```python
from build123d import *

# Parameters (mm, degrees)
SKETCH1_W           = 200
SKETCH1_H           = 200
BOSS_EXTRUDE1_DEPTH = 5
SKETCH2_W           = 100
SKETCH2_H           = 100
CUT_EXTRUDE1_DEPTH  = 10
FILLET1_R           = 10
FILLET2_R           = 10
SKETCH3_R           = 3
CUT_EXTRUDE2_DEPTH  = 10
SKETCH4_R           = 1.5
CUT_EXTRUDE3_DEPTH  = 10
SKETCH5_W           = 210
SKETCH5_H           = 210
BOSS_EXTRUDE2_DEPTH = 5
FILLET3_R           = 10
CIRPATTERN1_COUNT   = 4
SKETCH6_OUTSIDE_W   = 271.406
SKETCH6_OUTSIDE_H   = 271.406
SKETCH6_OUTSIDE_W_2 = 55
SKETCH6_OUTSIDE_H_2 = 132
CUT_EXTRUDE4_DEPTH  = 10
SKETCH8_W           = 55
SKETCH8_H           = 30
BOSS_EXTRUDE3_DEPTH = 5
SKETCH9_R           = 3
CUT_EXTRUDE6_DEPTH  = 5
SKETCH11_W          = 55
SKETCH11_H          = 19
CUT_EXTRUDE7_DEPTH  = 39
FILLET6_R           = 5
SKETCH12_W          = 15
SKETCH12_H          = 75
CUT_EXTRUDE8_DEPTH  = 10
FILLET7_R           = 5


with BuildPart() as part:
    # Sketch1 → Boss-Extrude1 (new body)
    with BuildSketch(Plane(origin=(0, 0, 0), x_dir=(1, 0, 0), z_dir=(0, 1, 0))):
        with Locations((100, 100)):
            Rectangle(SKETCH1_W, SKETCH1_H)
    extrude(amount=BOSS_EXTRUDE1_DEPTH)

    # Sketch2 → Cut-Extrude1 (cut)
    with BuildSketch(Plane(origin=(0, 5, 0), x_dir=(1, 0, 0), z_dir=(0, 1, 0))):
        with Locations((100, 100)):
            Rectangle(SKETCH2_W, SKETCH2_H)
    extrude(amount=-CUT_EXTRUDE1_DEPTH, mode=Mode.SUBTRACT)

    # Fillet1
    fillet1_edges = [part.edges().sort_by_distance(p)[0] for p in [
        (150, 2.5, -150),
        (150, 2.5, -50),
        (50, 2.5, -50),
        (50, 2.5, -150),
    ]]
    fillet(fillet1_edges, radius=FILLET1_R)

    # Fillet2
    fillet2_edges = [part.edges().sort_by_distance(p)[0] for p in [
        (0, 2.5, -200),
        (200, 2.5, -200),
        (200, 2.5, 0),
        (0, 2.5, 0),
    ]]
    fillet(fillet2_edges, radius=FILLET2_R)

    # Sketch3 → Cut-Extrude2 (cut)
    with BuildSketch(Plane(origin=(0, 5, 0), x_dir=(1, 0, 0), z_dir=(0, 1, 0))):
        with Locations((10, 190)):
            Circle(SKETCH3_R)
        with Locations((190, 190)):
            Circle(SKETCH3_R)
        with Locations((190, 10)):
            Circle(SKETCH3_R)
        with Locations((10, 10)):
            Circle(SKETCH3_R)
    extrude(amount=-CUT_EXTRUDE2_DEPTH, mode=Mode.SUBTRACT)

    # Sketch4 → Cut-Extrude3 (cut)
    with BuildSketch(Plane(origin=(0, 5, 0), x_dir=(1, 0, 0), z_dir=(0, 1, 0))):
        with Locations((198, 126)):
            Circle(SKETCH4_R)
        with Locations((191, 126)):
            Circle(SKETCH4_R)
        with Locations((196.89, 142)):
            Circle(SKETCH4_R)
        with Locations((154.75, 48)):
            Circle(SKETCH4_R)
        with Locations((196.75, 48)):
            Circle(SKETCH4_R)
        with Locations((196.75, 24)):
            Circle(SKETCH4_R)
        with Locations((154.75, 24)):
            Circle(SKETCH4_R)
        with Locations((242.150033952, -166.330778193)):
            Circle(SKETCH4_R)
        with Locations((285.400033952, -64.330778193)):
            Circle(SKETCH4_R)
        with Locations((242.150033952, -142.330778193)):
            Circle(SKETCH4_R)
        with Locations((284.290033952, -48.330778193)):
            Circle(SKETCH4_R)
        with Locations((284.150033952, -142.330778193)):
            Circle(SKETCH4_R)
        with Locations((284.150033952, -166.330778193)):
            Circle(SKETCH4_R)
        with Locations((278.400033952, -64.330778193)):
            Circle(SKETCH4_R)
    cut_extrude3 = extrude(amount=-CUT_EXTRUDE3_DEPTH, mode=Mode.SUBTRACT)

    # Sketch5 → Boss-Extrude2 (add)
    with BuildSketch(Plane(origin=(0, 5, 0), x_dir=(1, 0, 0), z_dir=(0, 1, 0))):
        with Locations((100, 100)):
            Rectangle(SKETCH5_W, SKETCH5_H)
        with BuildLine():
            Line((0, 190), (0, 10))
            ThreePointArc((0, 10), (2.928932188, 2.928932188), (10, 0))
            Line((10, 0), (190, 0))
            ThreePointArc((190, 0), (197.071067812, 2.928932188), (200, 10))
            Line((200, 10), (200, 190))
            ThreePointArc((200, 190), (197.071067812, 197.071067812), (190, 200))
            Line((190, 200), (10, 200))
            ThreePointArc((10, 200), (2.928932188, 197.071067812), (0, 190))
        make_face(mode=Mode.SUBTRACT)
    extrude(amount=-BOSS_EXTRUDE2_DEPTH)

    # Fillet3
    fillet3_edges = [part.edges().sort_by_distance(p)[0] for p in [
        (205, 2.5, -205),
        (205, 2.5, 5),
        (-5, 2.5, 5),
        (-5, 2.5, -205),
    ]]
    fillet(fillet3_edges, radius=FILLET3_R)

    # CirPattern1: Cut-Extrude3 ×4 about axis
    cirpattern1_axis = Axis((100, 0, -100), (0, 1, 0))
    for i in range(1, CIRPATTERN1_COUNT):
        add(cut_extrude3.rotate(cirpattern1_axis, i * 360 / CIRPATTERN1_COUNT), mode=Mode.SUBTRACT)

    # Sketch6 outside → Cut-Extrude4 (cut)
    with BuildSketch(Plane(origin=(0, 5, 0), x_dir=(1, 0, 0), z_dir=(0, 1, 0))):
        with Locations((100, 100)):
            Rectangle(SKETCH6_OUTSIDE_W, SKETCH6_OUTSIDE_H)
        with Locations((177.5, 83)):
            Rectangle(SKETCH6_OUTSIDE_W_2, SKETCH6_OUTSIDE_H_2, mode=Mode.SUBTRACT)
    extrude(amount=-CUT_EXTRUDE4_DEPTH, mode=Mode.SUBTRACT)

    # Sketch8 → Boss-Extrude3 (add)
    with BuildSketch(Plane(origin=(0, 5, 0), x_dir=(1, 0, 0), z_dir=(0, 1, 0))):
        with Locations((177.5, 2)):
            Rectangle(SKETCH8_W, SKETCH8_H)
        with Locations((177.5, 164)):
            Rectangle(SKETCH8_W, SKETCH8_H)
    extrude(amount=-BOSS_EXTRUDE3_DEPTH)

    # Sketch9 → Cut-Extrude6 (cut)
    with BuildSketch(Plane(origin=(0, 5, 0), x_dir=(1, 0, 0), z_dir=(0, 1, 0))):
        with Locations((177.5, 153.77)):
            Circle(SKETCH9_R)
        with Locations((177.5, -6.23)):
            Circle(SKETCH9_R)
    extrude(amount=-CUT_EXTRUDE6_DEPTH, mode=Mode.SUBTRACT)

    # Sketch11 → Cut-Extrude7 (cut)
    with BuildSketch(Plane(origin=(0, 5, 0), x_dir=(1, 0, 0), z_dir=(0, 1, 0))):
        with Locations((177.5, 169.5)):
            Rectangle(SKETCH11_W, SKETCH11_H)
    extrude(amount=-CUT_EXTRUDE7_DEPTH, mode=Mode.SUBTRACT)

    # Fillet6
    fillet6_edges = [part.edges().sort_by_distance(p)[0] for p in [
        (205, 2.5, 13),
        (150, 2.5, 13),
        (150, 2.5, -160),
        (205, 2.5, -160),
    ]]
    fillet(fillet6_edges, radius=FILLET6_R)

    # Sketch12 → Cut-Extrude8 (cut)
    with BuildSketch(Plane(origin=(0, 5, 0), x_dir=(1, 0, 0), z_dir=(0, 1, 0))):
        with Locations((157.5, 99.5)):
            Rectangle(SKETCH12_W, SKETCH12_H)
    extrude(amount=-CUT_EXTRUDE8_DEPTH, mode=Mode.SUBTRACT)

    # Fillet7
    fillet7_edges = [part.edges().sort_by_distance(p)[0] for p in [
        (150, 2.5, -62),
        (150, 2.5, -137),
        (165, 2.5, -137),
        (165, 2.5, -62),
    ]]
    fillet(fillet7_edges, radius=FILLET7_R)


solid = part.part
```
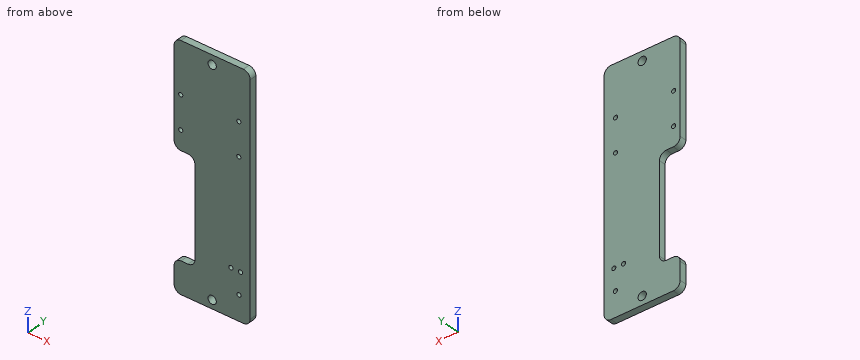
The listing builds one solid part. Answer for the finished solid, in the listing's coordinates (mm). Give positions to 0.01 mm unless a question says otherwise; leave off trailing zeros. Loops run counter-clockwise (first coordinate to the right, second up) from the corner with the lowest first, then second, coordinate; pieces in that order, holes last. Notation, with made-up numbers: (1, 79) - (52, 79) arc R31 ccw to (52, 108) - close; hole circle Ø6 at (-19.75, 28.5). An arc over 180 degrees is marked (long way). Return JSON: item names as keys, results as strings. Group by question number.
1. Find section D-D (x = 177). Write down the section's boundary in (y, z).
2. Straight lines are drawn through the part: line 1 (Z direction, x = 155, y = 0.85); line 2 (Z direction, x = 191, y = 1.1); line 3 (Z direction, x = 160, y = 4.15). For each, find the intervals that lie inside material, in ascending order. Write a range as [from, to].
3. Find section A-A (z = -48). Write down the section's boundary in (x, y), then the cut area to 3 significant figures.
4. Given pin 1 Ø5 at (x, z) = (177.5, -153.77) entering from -Y; pin 2 Ø5 at (x, z) = (174, -90.5) entering from -Y, each flat-ended and moving along its own axis, determine where each tip first touches the part or whether it passes through.
5. Find section C-C (y = 1.65). State how many separate pieces and enclosed holes the cut face has, then the cut area to 3 significant figures.
6. Find section B-B (x = 191). Write down the section's boundary in (y, z), then the cut area to 3 significant figures.
Verdict:
{
 "1": {"outline": "(0, -160) - (5, -160) - (5, -156.73) - (0, -156.73) - close; (0, -150.81) - (5, -150.81) - (5, 3.27) - (0, 3.27) - close; (0, 9.19) - (5, 9.19) - (5, 13) - (0, 13) - close"},
 "2": {"line 1": "z = [-160, -137], [-62, -49.48], [-46.52, -25.48], [-22.52, 13]", "line 2": "z = [-160, -127.5], [-124.5, 13]", "line 3": "z = [-160, -137], [-62, 13]"},
 "3": {"outline": "(150, 0) - (153.25, 0) - (153.25, 5) - (150, 5) - close; (156.25, 0) - (195.25, 0) - (195.25, 5) - (156.25, 5) - close; (198.25, 0) - (205, 0) - (205, 5) - (198.25, 5) - close", "area": "245 mm^2"},
 "4": {"pin 1": "passes through", "pin 2": "stops at y = 0"},
 "5": {"separate pieces": "1", "enclosed holes": "9", "area": "8,260 mm^2"},
 "6": {"outline": "(0, -160) - (5, -160) - (5, -127.5) - (0, -127.5) - close; (0, -124.5) - (5, -124.5) - (5, 13) - (0, 13) - close", "area": "850 mm^2"}
}
